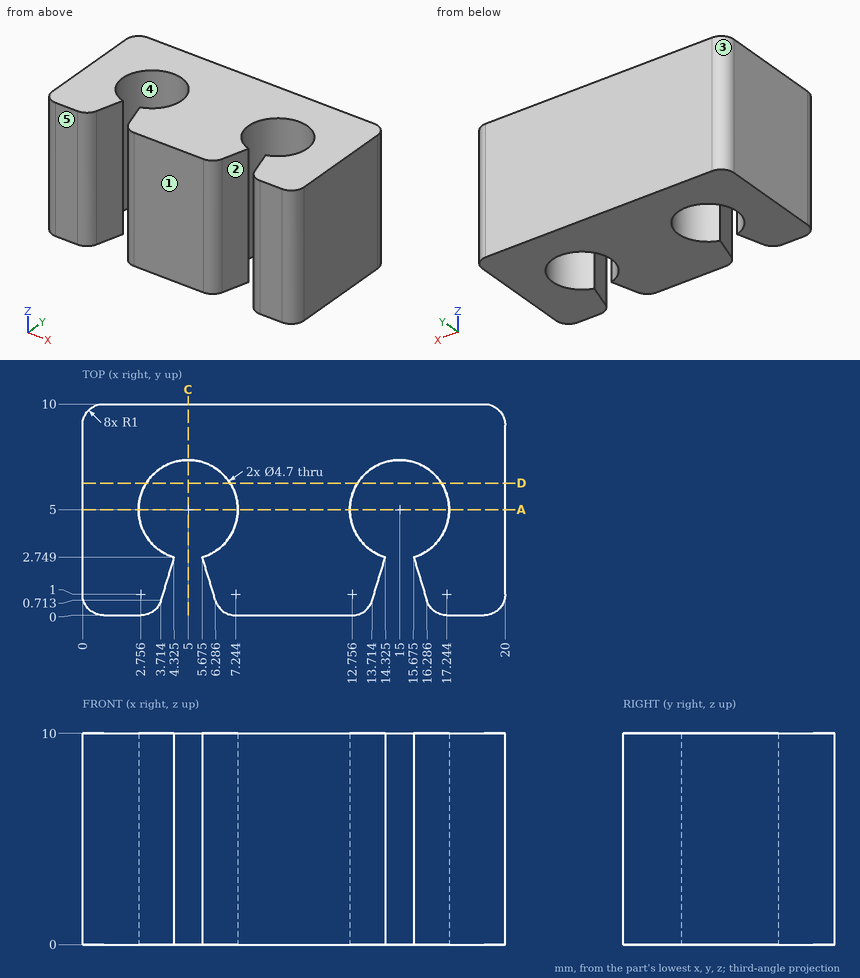
Design review of the part shown in the three views and the two pictorial views. Dimensions are in mm from the part's minimum x, y and z. A direction names the side the tool comes from. Round coordinates to 2 decimals unless told otherwise and drop trailing zeros. Order: outer loops, then holes, each group sorted by start corner. A loop starts at its lowest first (then second) coordinate and runs counter-clockwise, first axis right, second up. Notation, with made-up numbers: M -19,71 L 17,71 A22 cw 17,91 Z; hole C 51.25,-34 d3. An arc over 180 degrees is marked long. Put each result on its own line as item: value.
Q1. Consider section D-D (y = 6.25). State the section outline as (x, z) points.
Reported:
outline: M 0,0 L 3.01,0 L 3.01,10 L 0,10 Z; M 6.99,0 L 13.01,0 L 13.01,10 L 6.99,10 Z; M 16.99,0 L 20,0 L 20,10 L 16.99,10 Z
Q2. Draft analysis for pull direction X (two halves, no side actions). For the marked faces 3, 4 and 5, state which applies: released by +X, released by -X, zero draft, split by the parting line, or undercut.
Reported:
face 3: released by -X
face 4: undercut
face 5: zero draft
Q3. Machinability: for the marked faces 1 and 2, which of the approach directions +Z, -Z, +X, -X, +Y, -Y give a long, thin tool a straight path to every point of the face, cutting with its end or side? Answer none if there is none.
Reported:
face 1: +Z, -Z, +X, -X, -Y
face 2: +Z, -Z, -Y
Q4. Consider section A-A (y = 5). State the section outline as (x, z) points.
Reported:
outline: M 0,0 L 2.65,0 L 2.65,10 L 0,10 Z; M 7.35,0 L 12.65,0 L 12.65,10 L 7.35,10 Z; M 17.35,0 L 20,0 L 20,10 L 17.35,10 Z
Q5. Insertion check: pin 1 Ø3 at (x, z) = (5.5, 1) entering from -Y. The pin has a flat end and moves straight along its axis. Give the tip position at first contact, or say it passes through.
Reported:
pin 1: y = 0.03
Q6. To check wall thickness, follow line 1 (X direction, y = 5, z = 4); line 2 (X direction, y = 7, z = 7) (1 decimal); line 3 (Y direction, x = 5, z = 7.75). State the ranges of each line that lie inside material, in increasing order.
Reported:
line 1: 0 to 2.65, 7.35 to 12.65, 17.35 to 20
line 2: 0 to 3.8, 6.2 to 13.8, 16.2 to 20
line 3: 7.35 to 10
Q7. Consider section C-C (x = 5). State the section outline as (y, z) points.
Reported:
outline: M 7.35,0 L 10,0 L 10,10 L 7.35,10 Z
